The listing builds one solid part. Answer for the finished solid, in the listing's coordinates (mm). A direction names the side the tool comes from. Round coordinates to 2 decimals unless told otherwise and drop trailing zeros. Write each loop counter-clockwise with the first axis right and the second up, starting at its lowest first coordinate (ties: lowest second). Pieces come first, ordered by that corner, then holes. Notation, with made-up numbers: (-33.75, -22) - (5.25, -22) arc R23 ccw to (5.25, 11) - close; hole circle Ø10 at (87, -32). An arc over 180 degrees is marked (long way). Answer as CSV lines item,"result". Start each with the question number.
Item 1: Which of the six approach directions +Z, -Z, +X, -X, +Y, -Y give full straight-line access (tool end or side, diameter ignored) to faces 1 (the flat face through (65, 23.6, 2)), 2 (the flat face through (66.6, -1, 2)), 3 (the flat face through (33, -2.5, 2)), 4 (the flat face through (0, -1.17, 2)), 5 (the flat face through (63.1, 13, 2))?
Item 2: Straight lines are drawn through the part: line 1 along X through (y, z) = (18.5, 0.2); line 2 along Y through (x, z) = (0, 2); line 3 along X through (y, z) = (0, 1). For each, find the intervals that lie inside material, in ascending order. Write a range as [from, to].
Item 3: For a pull along X with two mould halves and no side action, classify faces 6 (the flat face through (-66.6, -1, 2)), 7 (the flat face through (-65, -25, 2)), 8 (the cylindrical face through (-0.04, 3.75, 1.73)) as pulls with the +X half, pulls with the -X half, needs draft (parallel to the pull), parting line crosses it, or undercut.
Item 4: A cutting plane is placed at A-A on x = 0. Determine the outline of the cut face in (y, z), and give its area (3 significant figures).
Item 5: Flat-ended cylindrical pins translate along their axes: pin 1 (1.3 mm diameter, centred on x = -67.5, y = 2, fed in from +Z); pin 2 (1 mm diameter, centred on y = -13, z = 2, fed in from -X); pin 3 (2 mm diameter, centred on x = -42, z = 0.5, fed in from +Y). Find the tip coordinate at first contact, or state that the pin passes through.
Item 6: A cutting plane is placed at B-B on y = -16.5. Determine the outline of the cut face in (x, z).
Item 7: A cutting plane is placed at C-C on z = 2.15. Determine the outline of the cut face in (x, y).
Item 8: A cutting plane is placed at D-D on y = 0. Determine the outline of the cut face in (x, z).
```python
from build123d import *

# Parameters (mm, degrees)
BOSS_EXTRUDE1_DEPTH = 3.5
SKETCH2_W           = 1.5
SKETCH2_H           = 2.3
CUT_EXTRUDE1_DEPTH  = 51
SKETCH3_W           = 136.2
SKETCH3_H           = 1.4
CUT_EXTRUDE2_DEPTH  = 4.5
FILLET1_R           = 0.3


with BuildPart() as part:
    # Sketch1 → Boss-Extrude1 (new body)
    with BuildSketch(Plane.XY):
        with BuildLine():
            Line((-63.1, 2.5), (-2.795084972, 2.5))
            ThreePointArc((-2.795084972, 2.5), (0, 3.75), (2.795084972, 2.5))
            Line((2.795084972, 2.5), (63.1, 2.5))
            Line((63.1, 2.5), (63.1, 25))
            Line((63.1, 25), (68.1, 25))
            Line((68.1, 25), (68.1, -25))
            Line((68.1, -25), (63.1, -25))
            Line((63.1, -25), (63.1, -2.5))
            Line((63.1, -2.5), (2.795084972, -2.5))
            ThreePointArc((2.795084972, -2.5), (0, -3.75), (-2.795084972, -2.5))
            Line((-2.795084972, -2.5), (-63.1, -2.5))
            Line((-63.1, -2.5), (-63.1, -25))
            Line((-63.1, -25), (-68.1, -25))
            Line((-68.1, -25), (-68.1, 25))
            Line((-68.1, 25), (-63.1, 25))
            Line((-63.1, 25), (-63.1, 2.5))
        make_face()
        with BuildLine():
            Line((-2.37773001, -1.17), (2.37773001, -1.17))
            ThreePointArc((2.37773001, -1.17), (0, 2.65), (-2.37773001, -1.17))
        make_face(mode=Mode.SUBTRACT)
    extrude(amount=BOSS_EXTRUDE1_DEPTH)

    # Sketch2 → Cut-Extrude1 (cut, through all)
    with BuildSketch(Plane.XZ.offset(25)):
        with Locations((67.35, 2.35)):
            Rectangle(SKETCH2_W, SKETCH2_H)
        with Locations((-67.35, 2.35)):
            Rectangle(SKETCH2_W, SKETCH2_H)
    extrude(amount=-CUT_EXTRUDE1_DEPTH, mode=Mode.SUBTRACT)

    # Sketch3 → Cut-Extrude2 (cut, through all)
    with BuildSketch(Plane.XY.offset(3.5)):
        with Locations((0, 24.3)):
            Rectangle(SKETCH3_W, SKETCH3_H)
    extrude(amount=-CUT_EXTRUDE2_DEPTH, mode=Mode.SUBTRACT)

    # Fillet1
    fillet1_edges = [part.edges().sort_by_distance(p)[0] for p in [
        (68.1, -0.7, 0),
        (-68.1, -0.7, 1.2),
        (68.1, -0.7, 1.2),
        (-68.1, -0.7, 0),
    ]]
    fillet(fillet1_edges, radius=FILLET1_R)


solid = part.part
```
Geometry says:
1,face 1,"+Z, -Z, +X, -X, +Y"
1,face 2,"+Z, +X, +Y, -Y"
1,face 3,"+Z, -Z, -Y"
1,face 4,"+Z, -Z"
1,face 5,"+Z, -Z, +Y"
2,line 1,"x = [-68.08, -63.1], [63.1, 68.08]"
2,line 2,"y = [-3.75, -1.17], [2.65, 3.75]"
2,line 3,"x = [-68.08, -2.65], [2.65, 68.08]"
3,face 6,"pulls with the -X half"
3,face 7,"needs draft"
3,face 8,"undercut"
4,outline,"(-3.75, 0) - (-1.17, 0) - (-1.17, 3.5) - (-3.75, 3.5) - close; (2.65, 0) - (3.75, 0) - (3.75, 3.5) - (2.65, 3.5) - close"
4,area,"12.9 mm^2"
5,pin 1,"stops at z = 1.2"
5,pin 2,"stops at x = -66.6"
5,pin 3,"stops at y = 2.5"
6,outline,"(-68.1, 0.3) arc R0.3 ccw to (-67.8, 0) - (-63.1, 0) - (-63.1, 3.5) - (-66.6, 3.5) - (-66.6, 1.2) - (-67.8, 1.2) arc R0.3 ccw to (-68.1, 0.9) - close; (63.1, 0) - (67.8, 0) arc R0.3 ccw to (68.1, 0.3) - (68.1, 0.9) arc R0.3 ccw to (67.8, 1.2) - (66.6, 1.2) - (66.6, 3.5) - (63.1, 3.5) - close"
7,outline,"(-66.6, -25) - (-63.1, -25) - (-63.1, -2.5) - (-2.8, -2.5) arc R3.75 ccw to (2.8, -2.5) - (63.1, -2.5) - (63.1, -25) - (66.6, -25) - (66.6, 23.6) - (63.1, 23.6) - (63.1, 2.5) - (2.8, 2.5) arc R3.75 ccw to (-2.8, 2.5) - (-63.1, 2.5) - (-63.1, 23.6) - (-66.6, 23.6) - close; hole (-2.38, -1.17) - (2.38, -1.17) arc R2.65 ccw (long way) to start"
8,outline,"(-68.1, 0.3) arc R0.3 ccw to (-67.8, 0) - (-2.65, 0) - (-2.65, 3.5) - (-66.6, 3.5) - (-66.6, 1.2) - (-67.8, 1.2) arc R0.3 ccw to (-68.1, 0.9) - close; (2.65, 0) - (67.8, 0) arc R0.3 ccw to (68.1, 0.3) - (68.1, 0.9) arc R0.3 ccw to (67.8, 1.2) - (66.6, 1.2) - (66.6, 3.5) - (2.65, 3.5) - close"
